from build123d import *

# Parameters (mm, degrees)
EXTRUDE_1_DEPTH     = 5
SKETCH_2_R          = 1.55
CUT_EXTRUDE_1_DEPTH = 234
EXTRUDE_3_DEPTH     = 3
SKETCH_4_W          = 188
SKETCH_4_H          = 10
EXTRUDE_4_DEPTH     = 5
SKETCH_5_W          = 70
SKETCH_5_H          = 46
EXTRUDE_5_DEPTH     = 5
EXTRUDE_6_DEPTH     = 4
CHAMFER_1_SIZE      = 10


with BuildPart() as part:
    # 草图1 → 凸台-拉伸1 (new, symmetric)
    with BuildSketch(Plane.XY):
        Polygon((-55.084006936, 98.602863112), (-7.242890373, -3.397136888), (0, 0), (-50, 106.602863112), (-70, 106.602863112), (-70, 98.602863112), align=None)
        Polygon((70, 106.602863112), (70, 98.602863112), (55.084006936, 98.602863112), (7.242890373, -3.397136888), (0, 0), (50, 106.602863112), align=None)
        Polygon((-70, -113.397136888), (-70, -105.397136888), (-55.084006936, -105.397136888), (-7.242890373, -3.397136888), (0, -6.794273777), (-50, -113.397136888), align=None)
        Polygon((55.084006936, -105.397136888), (7.242890373, -3.397136888), (0, -6.794273777), (50, -113.397136888), (70, -113.397136888), (70, -105.397136888), align=None)
        Polygon((-7.242890373, -3.397136888), (0, 0), (7.242890373, -3.397136888), align=None)
        Polygon((-7.242890373, -3.397136888), (7.242890373, -3.397136888), (0, -6.794273777), align=None)
    extrude(amount=EXTRUDE_1_DEPTH, both=True)

    # 草图2 → 切除-拉伸1 (cut)
    with BuildSketch(Plane(origin=(0, 106.602863112, 0), x_dir=(1, 0, 0), z_dir=(0, 1, 0))):
        with Locations(Location((-65, 0, 0), (0, 0, 180))):
            Circle(SKETCH_2_R)
        with Locations(Location((65, 0, 0), (0, 0, 180))):
            Circle(SKETCH_2_R)
    extrude(amount=-CUT_EXTRUDE_1_DEPTH, mode=Mode.SUBTRACT)

    # 草图3 → 凸台-拉伸3 (add, symmetric)
    with BuildSketch(Plane.XY):
        Polygon((8.660254038, 11.602863112), (-8.660254038, 11.602863112), (-17.320508076, -3.397136888), (-8.660254038, -18.397136888), (8.660254038, -18.397136888), (17.320508076, -3.397136888), align=None)
    extrude(amount=EXTRUDE_3_DEPTH, both=True)

    # 草图4 → 凸台-拉伸4 (add)
    with BuildSketch(Plane.XZ.offset(113.397136888)):
        Rectangle(SKETCH_4_W, SKETCH_4_H)
    extrude(amount=EXTRUDE_4_DEPTH)

    # 草图5 → 凸台-拉伸5 (add)
    with BuildSketch(Plane.XZ.offset(118.397136888)):
        with Locations((59, 28)):
            Rectangle(SKETCH_5_W, SKETCH_5_H)
        with Locations((-59, 28)):
            Rectangle(SKETCH_5_W, SKETCH_5_H)
    extrude(amount=-EXTRUDE_5_DEPTH)

    # 草图6 → 凸台-拉伸6 (add, symmetric)
    with BuildSketch(Plane.XY):
        Polygon((-31.163448655, 47.602863112), (-31.163448655, -54.397136888), (-37.163448655, -67.189480462), (-37.163448655, 60.395206685), align=None)
        Polygon((37.163448655, -67.189480462), (31.163448655, -54.397136888), (31.163448655, 47.602863112), (37.163448655, 60.395206685), align=None)
    extrude(amount=EXTRUDE_6_DEPTH, both=True)

    # 倒角1
    # the kernel refuses this chamfer: 10 mm, written as the material it adds along each edge
    with BuildSketch(Plane(origin=(-70, -113.397136888, 5), x_dir=(0, -0.0274958766105877, 0.9996219169112968), z_dir=(1, 0, 0))) as chamfer_1_piece_1_section:
        Polygon((CHAMFER_1_SIZE * 0.999621916911, -CHAMFER_1_SIZE * 0.0274958766106), (-CHAMFER_1_SIZE * 0.0274958766106, -CHAMFER_1_SIZE * 0.999621916911), (0, 0), align=None)
    chamfer_1_piece_1 = extrude(amount=45.71682988, mode=Mode.PRIVATE)
    chamfer_1_piece_1 = split(chamfer_1_piece_1, bisect_by=Plane(origin=(-58.48678517, -112.652054934, 8.358509751), z_dir=(-0.9053612966848448, 0.4246421110360305, 0)), keep=Keep.TOP, mode=Mode.PRIVATE)
    chamfer_1_piece_1 = split(chamfer_1_piece_1, bisect_by=Plane(origin=(-63.672942129, -105.397136888, 8.358509751), z_dir=(0, -1, 0)), keep=Keep.TOP, mode=Mode.PRIVATE)
    add(chamfer_1_piece_1)
    with BuildSketch(Plane(origin=(-70, -113.397136888, 5), x_dir=(0, -0.0274958766105877, 0.9996219169112968), z_dir=(1, 0, 0))) as chamfer_1_piece_2_section:
        Polygon((CHAMFER_1_SIZE * 0.999621916911, -CHAMFER_1_SIZE * 0.0274958766106), (-CHAMFER_1_SIZE * 0.0274958766106, -CHAMFER_1_SIZE * 0.999621916911), (0, 0), align=None)
    chamfer_1_piece_2 = extrude(amount=45.71682988, mode=Mode.PRIVATE)
    chamfer_1_piece_2 = split(chamfer_1_piece_2, bisect_by=Plane(origin=(-49.392291056, -112.10146662, 8.457184123), z_dir=(-0.9053612966848449, 0.42464211103603033, 0)), keep=Keep.TOP, mode=Mode.PRIVATE)
    chamfer_1_piece_2 = split(chamfer_1_piece_2, bisect_by=Plane(origin=(-56.635181429, -108.704329732, 8.457184123), z_dir=(0.9053612966848448, -0.4246421110360305, 0)), keep=Keep.TOP, mode=Mode.PRIVATE)
    chamfer_1_piece_2 = split(chamfer_1_piece_2, bisect_by=Plane(origin=(-53.013736242, -105.397136888, 8.457184123), z_dir=(0, -1, 0)), keep=Keep.TOP, mode=Mode.PRIVATE)
    add(chamfer_1_piece_2)
    with BuildSketch(Plane(origin=(-70, -113.397136888, 5), x_dir=(0, -0.0274958766105877, 0.9996219169112968), z_dir=(1, 0, 0))) as chamfer_1_piece_3_section:
        Polygon((CHAMFER_1_SIZE * 0.999621916911, -CHAMFER_1_SIZE * 0.0274958766106), (-CHAMFER_1_SIZE * 0.0274958766106, -CHAMFER_1_SIZE * 0.999621916911), (0, 0), align=None)
    chamfer_1_piece_3 = extrude(amount=45.71682988, mode=Mode.PRIVATE)
    chamfer_1_piece_3 = split(chamfer_1_piece_3, bisect_by=Plane(origin=(-46.659786315, -106.275610043, 5.402318693), z_dir=(-0.9053612966848449, 0.42464211103603033, 0)), keep=Keep.TOP, mode=Mode.PRIVATE)
    chamfer_1_piece_3 = split(chamfer_1_piece_3, bisect_by=Plane(origin=(-53.902676688, -102.878473155, 5.402318693), z_dir=(0.9053612966848448, -0.4246421110360305, 0)), keep=Keep.TOP, mode=Mode.PRIVATE)
    chamfer_1_piece_3 = split(chamfer_1_piece_3, bisect_by=Plane(origin=(-50.281231501, -105.397136888, 5.402318693), z_dir=(0, 1, 0)), keep=Keep.TOP, mode=Mode.PRIVATE)
    add(chamfer_1_piece_3)
    with BuildSketch(Plane(origin=(70, -113.397136888, 5), x_dir=(0, -0.027495876610584936, 0.9996219169112968), z_dir=(-1, 0, 0))) as chamfer_1_piece_4_section:
        Polygon((CHAMFER_1_SIZE * 0.999621916911, CHAMFER_1_SIZE * 0.0274958766106), (-CHAMFER_1_SIZE * 0.0274958766106, CHAMFER_1_SIZE * 0.999621916911), (0, 0), align=None)
    chamfer_1_piece_4 = extrude(amount=45.71682988, mode=Mode.PRIVATE)
    chamfer_1_piece_4 = split(chamfer_1_piece_4, bisect_by=Plane(origin=(63.672942129, -105.397136888, 8.358509751), z_dir=(0, -1, 0)), keep=Keep.TOP, mode=Mode.PRIVATE)
    chamfer_1_piece_4 = split(chamfer_1_piece_4, bisect_by=Plane(origin=(58.48678517, -112.652054934, 8.358509751), z_dir=(0.905361296684845, 0.4246421110360303, 0)), keep=Keep.TOP, mode=Mode.PRIVATE)
    add(chamfer_1_piece_4)
    with BuildSketch(Plane(origin=(70, -113.397136888, 5), x_dir=(0, -0.027495876610584936, 0.9996219169112968), z_dir=(-1, 0, 0))) as chamfer_1_piece_5_section:
        Polygon((CHAMFER_1_SIZE * 0.999621916911, CHAMFER_1_SIZE * 0.0274958766106), (-CHAMFER_1_SIZE * 0.0274958766106, CHAMFER_1_SIZE * 0.999621916911), (0, 0), align=None)
    chamfer_1_piece_5 = extrude(amount=45.71682988, mode=Mode.PRIVATE)
    chamfer_1_piece_5 = split(chamfer_1_piece_5, bisect_by=Plane(origin=(49.392291056, -112.10146662, 8.457184123), z_dir=(0.9053612966848449, 0.4246421110360304, 0)), keep=Keep.TOP, mode=Mode.PRIVATE)
    chamfer_1_piece_5 = split(chamfer_1_piece_5, bisect_by=Plane(origin=(53.013736242, -105.397136888, 8.457184123), z_dir=(0, -1, 0)), keep=Keep.TOP, mode=Mode.PRIVATE)
    chamfer_1_piece_5 = split(chamfer_1_piece_5, bisect_by=Plane(origin=(56.635181429, -108.704329732, 8.457184123), z_dir=(-0.905361296684845, -0.4246421110360303, 0)), keep=Keep.TOP, mode=Mode.PRIVATE)
    add(chamfer_1_piece_5)
    with BuildSketch(Plane(origin=(70, -113.397136888, 5), x_dir=(0, -0.027495876610584936, 0.9996219169112968), z_dir=(-1, 0, 0))) as chamfer_1_piece_6_section:
        Polygon((CHAMFER_1_SIZE * 0.999621916911, CHAMFER_1_SIZE * 0.0274958766106), (-CHAMFER_1_SIZE * 0.0274958766106, CHAMFER_1_SIZE * 0.999621916911), (0, 0), align=None)
    chamfer_1_piece_6 = extrude(amount=45.71682988, mode=Mode.PRIVATE)
    chamfer_1_piece_6 = split(chamfer_1_piece_6, bisect_by=Plane(origin=(46.659786315, -106.275610043, 5.402318693), z_dir=(0.9053612966848449, 0.4246421110360304, 0)), keep=Keep.TOP, mode=Mode.PRIVATE)
    chamfer_1_piece_6 = split(chamfer_1_piece_6, bisect_by=Plane(origin=(50.281231501, -105.397136888, 5.402318693), z_dir=(0, 1, 0)), keep=Keep.TOP, mode=Mode.PRIVATE)
    chamfer_1_piece_6 = split(chamfer_1_piece_6, bisect_by=Plane(origin=(53.902676688, -102.878473155, 5.402318693), z_dir=(-0.905361296684845, -0.4246421110360303, 0)), keep=Keep.TOP, mode=Mode.PRIVATE)
    add(chamfer_1_piece_6)
    with BuildSketch(Plane(origin=(70, -113.397136888, 5), x_dir=(0.9996219169112964, -0.02749587661059736, 0), z_dir=(0, 0, -1))) as chamfer_1_piece_7_section:
        Polygon((CHAMFER_1_SIZE * 0.999621916911, -CHAMFER_1_SIZE * 0.0274958766106), (-CHAMFER_1_SIZE * 0.0274958766106, -CHAMFER_1_SIZE * 0.999621916911), (0, 0), align=None)
    chamfer_1_piece_7 = extrude(amount=10, mode=Mode.PRIVATE)
    chamfer_1_piece_7 = split(chamfer_1_piece_7, bisect_by=Plane(origin=(73.457184123, -105.397136888, 0), z_dir=(0, -1, 0)), keep=Keep.TOP, mode=Mode.PRIVATE)
    add(chamfer_1_piece_7)
    with BuildSketch(Plane(origin=(-70, -113.397136888, -5), x_dir=(-0.9996219169112968, -0.027495876610586317, 0), z_dir=(0, 0, 1))) as chamfer_1_piece_8_section:
        Polygon((CHAMFER_1_SIZE * 0.999621916911, -CHAMFER_1_SIZE * 0.0274958766106), (-CHAMFER_1_SIZE * 0.0274958766106, -CHAMFER_1_SIZE * 0.999621916911), (0, 0), align=None)
    chamfer_1_piece_8 = extrude(amount=10, mode=Mode.PRIVATE)
    chamfer_1_piece_8 = split(chamfer_1_piece_8, bisect_by=Plane(origin=(-73.457184123, -105.397136888, 0), z_dir=(0, -1, 0)), keep=Keep.TOP, mode=Mode.PRIVATE)
    add(chamfer_1_piece_8)
    with BuildSketch(Plane(origin=(-70, -113.397136888, -5), x_dir=(-0.9996219169112968, -0.027495876610586317, 0), z_dir=(0, 0, 1))) as chamfer_1_piece_9a_section:
        Polygon((CHAMFER_1_SIZE * 0.999621916911, -CHAMFER_1_SIZE * 0.0274958766106), (-CHAMFER_1_SIZE * 0.0274958766106, -CHAMFER_1_SIZE * 0.999621916911), (0, 0), align=None)
    chamfer_1_piece_9a = extrude(amount=35.71682988, mode=Mode.PRIVATE)
    chamfer_1_piece_9a = split(chamfer_1_piece_9a, bisect_by=Plane(origin=(-73.457184123, -105.397136888, 17.85841494), z_dir=(0, -1, 0)), keep=Keep.TOP, mode=Mode.PRIVATE)
    chamfer_1_piece_9a = split(chamfer_1_piece_9a, bisect_by=Plane(origin=(-73.457184123, -110.402898176, 5), z_dir=(0, 0, 1)), keep=Keep.TOP, mode=Mode.PRIVATE)
    with BuildSketch(Plane(origin=(-95.71682988, -113.397136888, 5), x_dir=(0, -0.027495876610586317, 0.9996219169112968), z_dir=(1, 0, 0))) as chamfer_1_piece_9b_section:
        Polygon((CHAMFER_1_SIZE * 0.999621916911, -CHAMFER_1_SIZE * 0.0274958766106), (-CHAMFER_1_SIZE * 0.0274958766106, -CHAMFER_1_SIZE * 0.999621916911), (0, 0), align=None)
    chamfer_1_piece_9b = extrude(amount=71.433659759, mode=Mode.PRIVATE)
    chamfer_1_piece_9b = split(chamfer_1_piece_9b, bisect_by=Plane(origin=(-94, -110.402898176, 8.457184123), z_dir=(1, 0, 0)), keep=Keep.TOP, mode=Mode.PRIVATE)
    chamfer_1_piece_9b = split(chamfer_1_piece_9b, bisect_by=Plane(origin=(-82, -105.397136888, 8.457184123), z_dir=(0, -1, 0)), keep=Keep.TOP, mode=Mode.PRIVATE)
    chamfer_1_piece_9b = split(chamfer_1_piece_9b, bisect_by=Plane(origin=(-70, -110.402898176, 8.457184123), z_dir=(-1, 0, 0)), keep=Keep.TOP, mode=Mode.PRIVATE)
    chamfer_1_piece_9 = chamfer_1_piece_9a & chamfer_1_piece_9b
    add(chamfer_1_piece_9)
    with BuildSketch(Plane(origin=(70, -113.397136888, 30.71682988), x_dir=(0.9996219169112968, -0.0274958766105877, 0), z_dir=(0, 0, -1))) as chamfer_1_piece_10a_section:
        Polygon((CHAMFER_1_SIZE * 0.999621916911, -CHAMFER_1_SIZE * 0.0274958766106), (-CHAMFER_1_SIZE * 0.0274958766106, -CHAMFER_1_SIZE * 0.999621916911), (0, 0), align=None)
    chamfer_1_piece_10a = extrude(amount=35.71682988, mode=Mode.PRIVATE)
    chamfer_1_piece_10a = split(chamfer_1_piece_10a, bisect_by=Plane(origin=(73.457184123, -105.397136888, 17.85841494), z_dir=(0, -1, 0)), keep=Keep.TOP, mode=Mode.PRIVATE)
    chamfer_1_piece_10a = split(chamfer_1_piece_10a, bisect_by=Plane(origin=(73.457184123, -110.402898176, 5), z_dir=(0, 0, 1)), keep=Keep.TOP, mode=Mode.PRIVATE)
    with BuildSketch(Plane(origin=(95.71682988, -113.397136888, 5), x_dir=(0, -0.027495876610586317, 0.9996219169112968), z_dir=(-1, 0, 0))) as chamfer_1_piece_10b_section:
        Polygon((CHAMFER_1_SIZE * 0.999621916911, CHAMFER_1_SIZE * 0.0274958766106), (-CHAMFER_1_SIZE * 0.0274958766106, CHAMFER_1_SIZE * 0.999621916911), (0, 0), align=None)
    chamfer_1_piece_10b = extrude(amount=71.433659759, mode=Mode.PRIVATE)
    chamfer_1_piece_10b = split(chamfer_1_piece_10b, bisect_by=Plane(origin=(94, -110.402898176, 8.457184123), z_dir=(-1, 0, 0)), keep=Keep.TOP, mode=Mode.PRIVATE)
    chamfer_1_piece_10b = split(chamfer_1_piece_10b, bisect_by=Plane(origin=(70, -110.402898176, 8.457184123), z_dir=(1, 0, 0)), keep=Keep.TOP, mode=Mode.PRIVATE)
    chamfer_1_piece_10b = split(chamfer_1_piece_10b, bisect_by=Plane(origin=(82, -105.397136888, 8.457184123), z_dir=(0, -1, 0)), keep=Keep.TOP, mode=Mode.PRIVATE)
    chamfer_1_piece_10 = chamfer_1_piece_10a & chamfer_1_piece_10b
    add(chamfer_1_piece_10)


solid = part.part
Here's how the part is built. I have some questions about the finished solid (model axes, mm). A direction names the side the tool comes from. Give positions to 0.01 mm unless a question says otherwise; leave off trailing zeros. Order: outer loops, then holes, each group sorted by start corner. A loop starts at its lowest first (then second) coordinate and runs counter-clockwise, first axis right, second up. Notation, with made-up numbers: M -20.5,27.5 L 16.5,27.5 A14 ccw 16.5,39.5 Z; hole C -22,-7 d10. An arc over 180 degrees is marked long. Answer as a JSON object with one key per item and string values. Group by question number.
1) Please list where these lines run through material, in increasing order: L1, parallel to Z at x = 65, y = -110; L2, parallel to Z at x = -65, y = 101.75; L3, parallel to Y at x = 41, z = 29. Write a range as [from, to].
2) Suppose I cut it at C-C, the plane y = -50. Write out the boundary of the cut face in (x, z), plus the area to 3 significant figures.
3) We'd pull the mould along X, two halves only. Please class faces 1 (the flat face through (-63, -105.397, 1)), 2 (the flat face through (94, -116, 23)), 3 (the flat face through (-1.3, -113.397, 4.7)): pulls with the +X half, pulls with the -X half, needs draft (parallel to the pull), parting line crosses it, or undercut.
4) I'm going to push flat-ended pins straight in: pin 1 Ø3 at (x, z) = (65, 0) entering from +Y; pin 2 Ø1.8 at (x, y) = (35, 11) entering from +Z; pin 3 Ø6.5 at (y, z) = (-30, 2) entering from +X. Where does each tip first touch, or does it pass through?
5) Suppose I cut it at B-B, the plane y = 65. Write out the boundary of the cut face in (x, z), plus the area to 3 significant figures.
6) Suppose I cut it at A-A, the plane z = 24. Write out the boundary of the cut face in (x, y), plus the area to 3 significant figures.
7) On a 3-axis mill with a long thin cutter (end or side, diameter ignored), from which of +Z, -Z, +X, -X, +Y, -Y can I reach the whole of each face in a straight line? I mean faces 4 (the flat face through (-12, -3, -3)), 5 (the flat face through (-34, -3, 4)), 6 (the flat face through (63, 98.603, 0)). Say none if no direction works.
Results found:
{
 "1": {"L1": "[-5, -1.55], [1.55, 11.6]", "L2": "[-5, -1.55], [1.55, 5]", "L3": "[-118.4, -113.4]"},
 "2": {"outline": "M -37.16,-4 L -31.16,-4 L -31.16,4 L -37.16,4 Z; M -29.1,-5 L -20.26,-5 L -20.26,5 L -29.1,5 Z; M 20.26,-5 L 29.1,-5 L 29.1,5 L 20.26,5 Z; M 31.16,-4 L 37.16,-4 L 37.16,4 L 31.16,4 Z", "area": "273 mm²"},
 "3": {"face 1": "needs draft", "face 2": "pulls with the +X half", "face 3": "undercut"},
 "4": {"pin 1": "y = -113.4", "pin 2": "z = 4", "pin 3": "x = 37.16"},
 "5": {"outline": "M -39.32,-5 L -30.49,-5 L -30.49,5 L -39.32,5 Z; M 30.49,-5 L 39.32,-5 L 39.32,5 L 30.49,5 Z", "area": "177 mm²"},
 "6": {"outline": "M -94,-118.4 L -24,-118.4 L -24,-113.4 L -94,-113.4 Z; M 24,-118.4 L 94,-118.4 L 94,-113.4 L 24,-113.4 Z", "area": "700 mm²"},
 "7": {"face 4": "-Z", "face 5": "+Z, -X", "face 6": "+Z, -Z, +X"}
}
